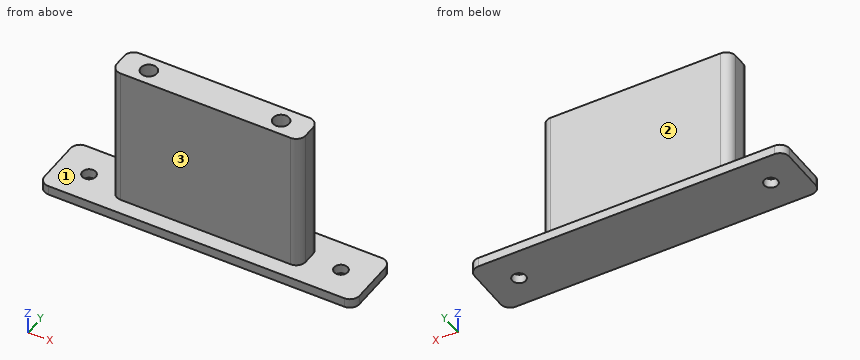
from build123d import *

# Parameters (mm, degrees)
SKETCH1_W           = 100
SKETCH1_H           = 20
SKETCH1_R           = 2.15
SKETCH1_R_2         = 2.55
BOSS_EXTRUDE1_DEPTH = 3
SKETCH2_R           = 2.55
BOSS_EXTRUDE3_DEPTH = 3
SKETCH3_W           = 60
SKETCH3_H           = 10
BOSS_EXTRUDE4_DEPTH = 45
SKETCH4_R           = 2.55
CUT_EXTRUDE3_DEPTH  = 8
FILLET1_R           = 3


with BuildPart() as part:
    # Sketch1 → Boss-Extrude1 (new body)
    with BuildSketch(Plane.XY):
        with Locations((50, -10)):
            Rectangle(SKETCH1_W, SKETCH1_H)
        with Locations((10, -10)):
            Circle(SKETCH1_R, mode=Mode.SUBTRACT)
        with Locations((90, -10)):
            Circle(SKETCH1_R, mode=Mode.SUBTRACT)
        with Locations((29, -10)):
            Circle(SKETCH1_R_2, mode=Mode.SUBTRACT)
        with Locations((71, -10)):
            Circle(SKETCH1_R_2, mode=Mode.SUBTRACT)
    extrude(amount=BOSS_EXTRUDE1_DEPTH)

    # Sketch2 → Boss-Extrude3 (add)
    with BuildSketch(Plane.XY.offset(3)):
        with Locations((71, -10)):
            Circle(SKETCH2_R)
        with Locations((29, -10)):
            Circle(SKETCH2_R)
    extrude(amount=-BOSS_EXTRUDE3_DEPTH)

    # Sketch3 → Boss-Extrude4 (add)
    with BuildSketch(Plane.XY.offset(3)):
        with Locations((50, -10)):
            Rectangle(SKETCH3_W, SKETCH3_H)
    extrude(amount=BOSS_EXTRUDE4_DEPTH)

    # Sketch4 → Cut-Extrude3 (cut)
    with BuildSketch(Plane.XY.offset(48)):
        with Locations((71, -10)):
            Circle(SKETCH4_R)
        with Locations((29, -10)):
            Circle(SKETCH4_R)
    extrude(amount=-CUT_EXTRUDE3_DEPTH, mode=Mode.SUBTRACT)

    # Fillet1
    fillet1_edges = [part.edges().sort_by_distance(p)[0] for p in [
        (80, -15, 25.5),
        (80, -5, 25.5),
        (20, -5, 25.5),
        (20, -15, 25.5),
        (0, 0, 1.5),
        (100, 0, 1.5),
        (100, -20, 1.5),
        (0, -20, 1.5),
    ]]
    fillet(fillet1_edges, radius=FILLET1_R)


solid = part.part
Input: part model. Units: mm. Frame: model coordinates. Face numbers are marked on the shaded views. Coordinates: 2 decimals unless noted, no trailing zeros. Write each loop counter-clockwise with the first axis right and the second up, starting at its lowest first coordinate (ties: lowest second). Pieces come first, ordered by that corner, then holes. Notation, with made-up numbers: M 27.5,38.25 L 56.5,38.25 A21 ccw 56.5,65.25 Z; hole C 8.25,8 d1. An arc over 180 degrees is marked long. Answer as a JSON object with one key per item and string values. Group by question number.
(1) Contact query for flat-ended pins moving along their axis: P1, Ø13.5, axis at x = 54, z = 24.5, coming from the -Y side; P2, Ø4, axis at x = 30, z = 17, coming from the +Y side; P3, Ø1.5, axis at y = -7.5, z = 41, coming from the -X side; P4, Ø4, axis at x = 90, y = -10, coming from the +Z side. Output: stop coordinate, or through.
(2) Section D-D on x = 29. Output: boundary loops of the cut face in (y, z), plus the area to 3 significant figures.
(3) Section A-A on y = -10. Output: boundary loops of the cut face in (x, z).
(4) Mould query, pull axis Y, two halves, no side actions, for the marked faces 1, 2 and 3. Classes: pulls with the +Y half, pulls with the -Y half, needs draft (parallel to the pull), parting line crosses it, or undercut.
(5) Section B-B on x = 90. Output: boundary loops of the cut face in (y, z).
(6) Section C-C on z = 45. Output: boundary loops of the cut face in (x, y), plus the area to 3 significant figures.
(7) Ray query, line 1 along X through (y, z) = (-9, 45); line 2 along Y through (x, z) = (71, 45.5); line 3 along Y through (x, z) = (90, 0.7). Return the intervals inside material, ascending. Write a range as [from, to].
Result set:
{
 "1": {"P1": "stops at y = -15", "P2": "stops at y = -5", "P3": "stops at x = 20", "P4": "passes through"},
 "2": {"outline": "M -20,0 L 0,0 L 0,3 L -5,3 L -5,48 L -7.45,48 L -7.45,40 L -12.55,40 L -12.55,48 L -15,48 L -15,3 L -20,3 Z", "area": "469 mm2"},
 "3": {"outline": "M 0,0 L 7.85,0 L 7.85,3 L 0,3 Z; M 12.15,0 L 87.85,0 L 87.85,3 L 80,3 L 80,48 L 73.55,48 L 73.55,40 L 68.45,40 L 68.45,48 L 31.55,48 L 31.55,40 L 26.45,40 L 26.45,48 L 20,48 L 20,3 L 12.15,3 Z; M 92.15,0 L 100,0 L 100,3 L 92.15,3 Z"},
 "4": {"face 1": "needs draft", "face 2": "pulls with the +Y half", "face 3": "pulls with the -Y half"},
 "5": {"outline": "M -20,0 L -12.15,0 L -12.15,3 L -20,3 Z; M -7.85,0 L 0,0 L 0,3 L -7.85,3 Z"},
 "6": {"outline": "M 20,-12 A3 ccw 23,-15 L 77,-15 A3 ccw 80,-12 L 80,-8 A3 ccw 77,-5 L 23,-5 A3 ccw 20,-8 Z; hole C 29,-10 d5.1; hole C 71,-10 d5.1", "area": "551 mm2"},
 "7": {"line 1": "x = [20, 26.65], [31.35, 68.65], [73.35, 80]", "line 2": "y = [-15, -12.55], [-7.45, -5]", "line 3": "y = [-20, -12.15], [-7.85, 0]"}
}
